Build history of the part. All positions in model axes, mm. A direction names the side the tool comes from. Round coordinates to 2 decimals unless told otherwise and drop trailing zeros. Write each loop counter-clockwise with the first axis right and the second up, starting at its lowest first coordinate (ties: lowest second). Pieces come first, ordered by that corner, then holes.
1) Saw through at B-B (y = 15.75). Write the cut outline in (x, z), plus the area to 3 significant figures.
2) Saw through at A-A (x = 0). Write the cut outline in (y, z) (3 decimals), plus the area to 3 significant figures.
3) Flat gauge pins, fed straight in: pin 1 (1 mm diameter, centred on y = 15, z = -0.5, fed in from +X); pin 2 (0.6 mm diameter, centred on x = 0, y = 26.5, fed in from -Z) (3 decimals). Where does each tip first touch, or does it go through?
4) Which spindle directions (+Z, -Z, +X, -X, +Y, -Y) get a long thin tool onto all of the face, cutting with end or side? Do faces 1 (the flat face through (0, 27, 0)), 2 (the cylindrical face through (-0.506, 18.809, -0.323)), 3 (the cylindrical face through (-0.029, 25.844, 0.654)). Say none if no direction does.
5) Wall check: probe 1 along X at (y, z) = (14, 0); probe 2 along Y at (x, z) = (0.2, -0.1). Give the ranges that are in metal, low to high.
from build123d import *

# Parameters (mm, degrees)
CUT_EXTRUDE1_START = -1.25
CUT_EXTRUDE1_DEPTH = 1.25


with BuildPart() as part:
    # Sketch1 → Revolve1 (revolve)
    with BuildSketch(Plane.XY, mode=Mode.PRIVATE) as revolve1_sk:
        Polygon((0.6, 24.386414327), (0.6, 13.386414327), (0.35, 13.136414327), (0, 13.136414327), (0, 27.543335196), (0.655, 27.543335196), (0.655, 24.793335196), (0.85, 24.680751894), (0.85, 24.530751894), align=None)
    revolve(revolve1_sk.sketch.rotate(Axis((0, 0, 0), (0, 1, 0)), 90), axis=Axis((0, 0, 0), (0, 1, 0)))

    # Sketch2 → Cut-Extrude1 (cut)
    with BuildSketch(Plane(origin=(0, 27.543335196, 0), x_dir=(-1, 0, 0), z_dir=(0, 1, 0)).offset(CUT_EXTRUDE1_START)):
        with BuildLine():
            Line((-0.655, 0), (0.655, 0))
            ThreePointArc((0.655, 0), (0, -0.655), (-0.655, 0))
        make_face()
    extrude(amount=CUT_EXTRUDE1_DEPTH, mode=Mode.SUBTRACT)


solid = part.part
Evaluation:
1. outline: circle Ø1.2 at (0, 0)
1. area: 1.13 mm2
2. outline: (13.136, -0.35) - (13.386, -0.6) - (24.386, -0.6) - (24.531, -0.85) - (24.681, -0.85) - (24.793, -0.655) - (26.293, -0.655) - (26.293, 0) - (27.543, 0) - (27.543, 0.655) - (24.793, 0.655) - (24.681, 0.85) - (24.531, 0.85) - (24.386, 0.6) - (13.386, 0.6) - (13.136, 0.35) - close
2. area: 16.9 mm2
3. pin 1: stops at x = 0.6
3. pin 2: stops at z = -0.655
4. face 1: -Z, +X, -X, +Y
4. face 2: -Y
4. face 3: +Y
5. probe 1: x = -0.6 to 0.6
5. probe 2: y = 13.14 to 26.29
